```python
from build123d import *

# Parameters (mm, degrees)
BOSS_EXTRUDE1_DEPTH     = 5
BOSS_EXTRUDE2_DEPTH     = 7
SKETCH3_R               = 1.5
SKETCH3_W               = 8
SKETCH3_H               = 8
SKETCH3_R_2             = 2.5
BOSS_EXTRUDE3_DEPTH     = 5
SKETCH4_R               = 2.5
BOSS_EXTRUDE4_DEPTH     = 5
CUT_EXTRUDE1_DEPTH      = 123.769787834
CUT_EXTRUDE1_DEPTH_BACK = 123.769787834
SKETCH5_R               = 2.5
SKETCH5_R_2             = 2.55926668
SKETCH5_R_3             = 1.5
FILLET1_R               = 3.5


with BuildPart() as part:
    # Sketch1 → Boss-Extrude1 (new body)
    with BuildSketch(Plane(origin=(0, 0, 0), x_dir=(1, 0, 0), z_dir=(0, 1, 0))):
        Polygon((-57.597316241, 51.805869074), (-57.597316241, -8.444130926), (-46.097316241, -28.194130926), (-46.097316241, -108.194130926), (43.902683759, -108.194130926), (43.902683759, -28.194130926), (55.402683759, -8.444130926), (55.402683759, 51.805869074), align=None)
    extrude(amount=BOSS_EXTRUDE1_DEPTH)

    # Sketch2 → Boss-Extrude2 (add)
    with BuildSketch(Plane(origin=(0, 5, 0), x_dir=(1, 0, 0), z_dir=(0, 1, 0))):
        Polygon((-46.097316241, -28.194130926), (-46.097316241, -108.194130926), (43.902683759, -108.194130926), (43.902683759, -28.194130926), (41.402683759, -28.194130926), (41.402683759, -105.694130926), (-43.597316241, -105.694130926), (-43.597316241, -28.194130926), align=None)
        Polygon((52.902683759, -6.988434723), (55.402683759, -8.444130926), (43.902683759, -28.194130926), (41.402683759, -26.738434723), align=None)
        Polygon((41.402683759, -28.194130926), (43.902683759, -28.194130926), (41.402683759, -26.738434723), align=None)
        Polygon((52.902683759, -6.988434723), (55.402683759, -8.444130926), (55.402683759, -6.988434723), align=None)
        Polygon((-57.597316241, 51.805869074), (-57.597316241, -6.988434723), (-55.097316241, -6.988434723), (-55.097316241, 49.305869074), (52.902683759, 49.305869074), (52.902683759, -6.988434723), (55.402683759, -6.988434723), (55.402683759, 51.805869074), align=None)
        Polygon((-43.597316241, -26.738434723), (-46.097316241, -28.194130926), (-43.597316241, -28.194130926), align=None)
        Polygon((-43.597316241, -26.738434723), (-46.097316241, -28.194130926), (-57.597316241, -8.444130926), (-55.097316241, -6.988434723), align=None)
        Polygon((-57.597316241, -6.988434723), (-57.597316241, -8.444130926), (-55.097316241, -6.988434723), align=None)
    extrude(amount=BOSS_EXTRUDE2_DEPTH)

    # Sketch3 → Boss-Extrude3 (add)
    # profile 1 of 3: a face of its own
    with BuildSketch(Plane(origin=(0, 5, 0), x_dir=(1, 0, 0), z_dir=(0, 1, 0))):
        Polygon((-43.597316241, -99.694130926), (-43.597316241, -105.694130926), (41.402683759, -105.694130926), (41.402683759, -99.694130926), (32.902683759, -99.694130926), (20.902683759, -102.694130926), (-23.097316241, -102.694130926), (-35.097316241, -99.694130926), align=None)
        with Locations(Location((-39.347316241, -101.944130926, 0), (0, 0, 270))):
            Circle(SKETCH3_R, mode=Mode.SUBTRACT)
        with Locations(Location((37.152683759, -101.944130926, 0), (0, 0, 270))):
            Circle(SKETCH3_R, mode=Mode.SUBTRACT)
    # profile 2 of 3: a face of its own
    with BuildSketch(Plane(origin=(0, 5, 0), x_dir=(1, 0, 0), z_dir=(0, 1, 0))):
        with Locations((-51.097316241, 45.305869074)):
            Rectangle(SKETCH3_W, SKETCH3_H)
        with Locations(Location((-51.097316241, 45.305869074, 0), (0, 0, 270))):
            Circle(SKETCH3_R_2, mode=Mode.SUBTRACT)
    # profile 3 of 3: a face of its own
    with BuildSketch(Plane(origin=(0, 5, 0), x_dir=(1, 0, 0), z_dir=(0, 1, 0))):
        with Locations((48.902683759, 45.305869074)):
            Rectangle(SKETCH3_W, SKETCH3_H)
        with Locations(Location((48.902683759, 45.305869074, 0), (0, 0, 270))):
            Circle(SKETCH3_R_2, mode=Mode.SUBTRACT)
    extrude(amount=BOSS_EXTRUDE3_DEPTH)

    # Sketch4 → Boss-Extrude4 (add)
    # profile 1 of 2: a face of its own
    with BuildSketch(Plane(origin=(0, 5, 0), x_dir=(1, 0, 0), z_dir=(0, 1, 0))):
        Polygon((1.402683759, 10.130869074), (-55.097316241, 10.130869074), (-55.097316241, -6.988434723), (-43.597316241, -26.738434723), (-43.597316241, 0.130869074), (1.402683759, 0.130869074), align=None)
        with Locations(Location((-31.847316241, 5.130869074, 0), (0, 0, 90))):
            Circle(SKETCH4_R, mode=Mode.SUBTRACT)
        with Locations(Location((-21.847316241, 5.130869074, 0), (0, 0, 90))):
            Circle(SKETCH4_R, mode=Mode.SUBTRACT)
    # profile 2 of 2: a face of its own
    with BuildSketch(Plane(origin=(0, 5, 0), x_dir=(1, 0, 0), z_dir=(0, 1, 0))):
        Polygon((39.6145491, 10.130869074), (39.6145491, 0.130869074), (41.402683759, 0.130869074), (41.402683759, -26.738434723), (52.902683759, -6.988434723), (52.902683759, 10.130869074), align=None)
    extrude(amount=BOSS_EXTRUDE4_DEPTH)

    # Sketch5 → Cut-Extrude1 (cut, two sides: drawn at the far end of the back side and taken through both)
    with BuildSketch(Plane(origin=(0, 5, 0), x_dir=(1, 0, 0), z_dir=(0, 1, 0)).offset(-CUT_EXTRUDE1_DEPTH_BACK)):
        with Locations(Location((-21.847316241, 5.130869074, 0), (0, 0, 90))):
            Circle(SKETCH5_R)
        with Locations(Location((-31.847316241, 5.130869074, 0), (0, 0, 270))):
            Circle(SKETCH5_R_2)
        with Locations(Location((-39.347316241, -101.944130926, 0), (0, 0, 270))):
            Circle(SKETCH5_R_3)
        with Locations(Location((37.152683759, -101.944130926, 0), (0, 0, 270))):
            Circle(SKETCH5_R_3)
        with Locations(Location((-51.097316241, 45.305869074, 0), (0, 0, 270))):
            Circle(SKETCH5_R)
        with Locations(Location((48.902683759, 45.305869074, 0), (0, 0, 270))):
            Circle(SKETCH5_R)
        with Locations(Location((-49.597316241, -6.988434723, 0), (0, 0, 270))):
            Circle(SKETCH5_R)
        with Locations(Location((47.402683759, -6.988434723, 0), (0, 0, 270))):
            Circle(SKETCH5_R)
    extrude(amount=CUT_EXTRUDE1_DEPTH + CUT_EXTRUDE1_DEPTH_BACK, mode=Mode.SUBTRACT)

    # Fillet1
    # the kernel refuses this fillet: 3.5 mm, written as the material it adds along each edge
    with BuildSketch(Plane(origin=(41.402683759, 5, 99.694130926), x_dir=(0, 0, -1), z_dir=(0, 1, 0)), Plane(origin=(-55.097316241, 5, -41.305869074), x_dir=(0, 0, 1), z_dir=(0, 1, 0)), Plane(origin=(44.902683759, 5, -49.305869074), x_dir=(-1, 0, 0), z_dir=(0, 1, 0)), Plane(origin=(52.902683759, 5, -10.130869074), x_dir=(0, 0, -1), z_dir=(0, 1, 0)), Plane(origin=(-43.597316241, 5, -0.130869074), x_dir=(0, 0, 1), z_dir=(0, 1, 0))) as fillet1_piece_1:
        with BuildLine():
            CenterArc((FILLET1_R, FILLET1_R), FILLET1_R, 180, 90)
            Line((0, FILLET1_R), (0, 0))
            Line((0, 0), (FILLET1_R, 0))
        make_face()
    extrude(amount=5)
    with BuildSketch(Plane(origin=(20.902683759, 3.922825776, 102.694130926), x_dir=(-1, 0, 0), z_dir=(0, 1, 0)), Plane(origin=(-23.097316241, 3.922825776, 102.694130926), x_dir=(-0.9701425001453338, 0, -0.2425356250363252), z_dir=(0, 1, 0))) as fillet1_piece_2:
        with BuildLine():
            CenterArc((FILLET1_R * 0.123105625618, -FILLET1_R), FILLET1_R, 90, 14.036243468)
            Line((-FILLET1_R * 0.119429999419, -FILLET1_R * 0.0298574998547), (0, 0))
            Line((0, 0), (FILLET1_R * 0.123105625618, 0))
        make_face()
    extrude(amount=6.077174224)
    with BuildSketch(Plane(origin=(-43.597316241, 5, 99.694130926), x_dir=(0, 0, -1), z_dir=(0, 1, 0)), Plane(origin=(-47.097316241, 5, -49.305869074), x_dir=(1, 0, 0), z_dir=(0, 1, 0)), Plane(origin=(52.902683759, 5, -41.305869074), x_dir=(0, 0, 1), z_dir=(0, 1, 0)), Plane(origin=(-55.097316241, 5, -10.130869074), x_dir=(0, 0, -1), z_dir=(0, 1, 0))) as fillet1_piece_3:
        with BuildLine():
            CenterArc((FILLET1_R, -FILLET1_R), FILLET1_R, 90, 90)
            Line((0, -FILLET1_R), (0, 0))
            Line((0, 0), (FILLET1_R, 0))
        make_face()
    extrude(amount=5)
    with BuildSketch(Plane(origin=(43.902683759, 12, 28.194130926), x_dir=(0.5031907286678252, 0, -0.864175381842565), z_dir=(0, -1, 0)), Plane(origin=(-46.097316241, 0, 28.194130926), x_dir=(-0.5031907286678269, 0, -0.8641753818425641), z_dir=(0, 1, 0))) as fillet1_piece_4:
        with BuildLine():
            CenterArc((FILLET1_R * 0.269926710528, FILLET1_R), FILLET1_R, 239.788677614, 30.211322386)
            Line((-FILLET1_R * 0.23326401814, FILLET1_R * 0.135824618157), (0, 0))
            Line((0, 0), (FILLET1_R * 0.269926710528, 0))
        make_face()
    extrude(amount=12)
    with BuildSketch(Plane(origin=(41.402683759, 5, -0.130869074), x_dir=(0, 0, 1), z_dir=(0, 1, 0))) as fillet1_piece_5:
        with BuildLine():
            CenterArc((3.052788407, -3.5), FILLET1_R, 90, 60.718267745)
            Line((0, -1.788134659), (0, 0))
            Line((0, 0), (3.052788407, 0))
        make_face()
    extrude(amount=5)
    # the kernel refuses this fillet: 3.5 mm, written as the material it takes off along each edge
    with BuildSketch(Plane(origin=(32.902683759, 5, 99.694130926), x_dir=(1, 0, 0), z_dir=(0, 1, 0)), Plane(origin=(-35.097316241, 5, 99.694130926), x_dir=(0.9701425001453338, 0, 0.2425356250363252), z_dir=(0, 1, 0))) as fillet1_2_piece_1:
        with BuildLine():
            CenterArc((FILLET1_R * 0.123105625618, -FILLET1_R), FILLET1_R, 90, 14.036243468)
            Line((-FILLET1_R * 0.119429999419, -FILLET1_R * 0.0298574998547), (0, 0))
            Line((0, 0), (FILLET1_R * 0.123105625618, 0))
        make_face()
    extrude(amount=6.077174224, mode=Mode.SUBTRACT)
    with BuildSketch(Plane(origin=(-47.097316241, 5, -41.305869074), x_dir=(-1, 0, 0), z_dir=(0, 1, 0)), Plane(origin=(44.902683759, 5, -41.305869074), x_dir=(0, 0, -1), z_dir=(0, 1, 0)), Plane(origin=(39.6145491, 5, -10.130869074), x_dir=(1, 0, 0), z_dir=(0, 1, 0)), Plane(origin=(1.402683759, 5, -10.130869074), x_dir=(0, 0, 1), z_dir=(0, 1, 0))) as fillet1_2_piece_2:
        with BuildLine():
            CenterArc((FILLET1_R, -FILLET1_R), FILLET1_R, 90, 90)
            Line((0, -FILLET1_R), (0, 0))
            Line((0, 0), (FILLET1_R, 0))
        make_face()
    extrude(amount=13.75, mode=Mode.SUBTRACT)
    with BuildSketch(Plane(origin=(55.402683759, 14.361858717, 8.444130926), x_dir=(0, 0, -1), z_dir=(0, -1, 0)), Plane(origin=(-57.597316241, -2.361858717, 8.444130926), x_dir=(0, 0, -1), z_dir=(0, 1, 0))) as fillet1_2_piece_3:
        with BuildLine():
            CenterArc((FILLET1_R * 0.269926710528, -FILLET1_R), FILLET1_R, 90, 30.211322386)
            Line((-FILLET1_R * 0.23326401814, -FILLET1_R * 0.135824618157), (0, 0))
            Line((0, 0), (FILLET1_R * 0.269926710528, 0))
        make_face()
    extrude(amount=16.723717434, mode=Mode.SUBTRACT)
    with BuildSketch(Plane(origin=(43.902683759, 20.75, 108.194130926), x_dir=(-1, 0, 0), z_dir=(0, -1, 0))) as fillet1_2_piece_4:
        with BuildLine():
            CenterArc((FILLET1_R, FILLET1_R), FILLET1_R, 180, 90)
            Line((0, FILLET1_R), (0, 0))
            Line((0, 0), (FILLET1_R, 0))
        make_face()
    extrude(amount=29.5, mode=Mode.SUBTRACT)
    with BuildSketch(Plane(origin=(-46.097316241, -8.75, 108.194130926), x_dir=(0, 0, -1), z_dir=(0, 1, 0)), Plane(origin=(-57.597316241, -8.75, -51.805869074), x_dir=(1, 0, 0), z_dir=(0, 1, 0)), Plane(origin=(55.402683759, -8.75, -51.805869074), x_dir=(0, 0, 1), z_dir=(0, 1, 0))) as fillet1_2_piece_5:
        with BuildLine():
            CenterArc((FILLET1_R, -FILLET1_R), FILLET1_R, 90, 90)
            Line((0, -FILLET1_R), (0, 0))
            Line((0, 0), (FILLET1_R, 0))
        make_face()
    extrude(amount=29.5, mode=Mode.SUBTRACT)
    with BuildSketch(Plane(origin=(1.402683759, 5, -0.130869074), x_dir=(0, 0, -1), z_dir=(0, 1, 0))) as fillet1_2_piece_6:
        with BuildLine():
            CenterArc((FILLET1_R, FILLET1_R), FILLET1_R, 180, 90)
            Line((0, FILLET1_R), (0, 0))
            Line((0, 0), (FILLET1_R, 0))
        make_face()
    extrude(amount=13.75, mode=Mode.SUBTRACT)


solid = part.part
```
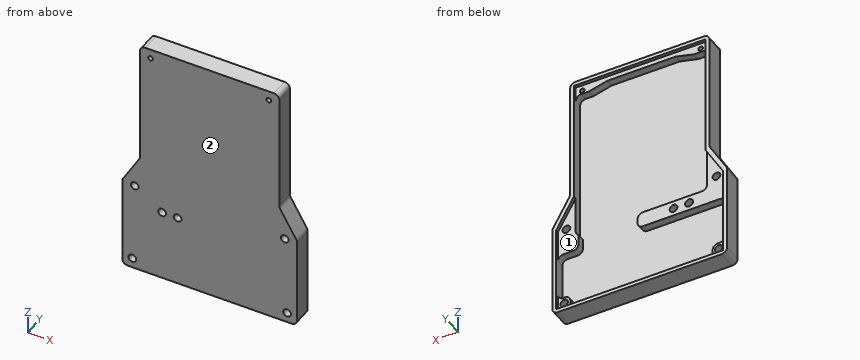
Input: part model. Units: mm. Frame: model coordinates. Face numbers are marked on the shaded views. Coordinates: 2 decimals unless noted, no trailing zeros. Loops run counter-clockwise (first coordinate to the right, second up) from the corner with the lowest first, then second, coordinate; pieces in that order, holes last. Notation, with made-up numbers: M -14,16.5 L 41,16.5 A21 cw 41,46.5 Z; hole C 77,-18 d4. An arc over 180 degrees is marked long. Use a Markdown table: item, result. Add a question column.
1) Section C-C, the plane z = 24.5. Return the cut outline in (x, y), plus the area to 3 significant figures.
2) Section B-B, the plane z = 73.5. Return the cut outline in (x, y).
3) Pin query (flat end, axial travel): P1, Ø5, axis at x = -8, z = 98.5, coming from the +Y side; P2, Ø1, axis at y = 3, z = 24, coming from the -X side; P3, Ø3.5, axis at x = 37.15, z = 101.94, coming from the +Y side; P4, Ø4.5, axis at x = -51.1, z = -45.31, coming from the +Y side. Return the tip coordinate at first contact, or that it passes through.
4) Section A-A, the plane y = 1.75. Give the number of separate pieces and of enclosed holes in the cut face, plus the area to 3 significant figures.
5) Draft query along X for the marked faces 1 and 2. Return one class per face: +X half, -X half, draft (parallel to the pull), parting line (faces both ways), or undercut.
6) Line query: L1, parallel to X at y = 6, z = -22.5; L2, parallel to X at y = 5.75, z = 39; L3, parallel to Z at x = 50.5, y = 7.25. Output: solid intervals per line, ascending. Write a range as from..to.
Answer below:
| question | item | result |
|---|---|---|
| 1 | outline | M -48.25,0 L 46.05,0 L 46.05,12 L 42.71,12 L 42.71,10 L 41.4,10 L 41.4,5 L -43.6,5 L -43.6,10 L -44.9,10 L -44.9,12 L -48.25,12 Z |
| 1 | area | 531 mm2 |
| 2 | outline | M -46.1,0 L 43.9,0 L 43.9,12 L 41.4,12 L 41.4,5 L -43.6,5 L -43.6,12 L -46.1,12 Z |
| 3 | P1 | y = 5 |
| 3 | P2 | x = -48.83 |
| 3 | P3 | y = 10 |
| 3 | P4 | through |
| 4 | separate pieces | 1 |
| 4 | enclosed holes | 8 |
| 4 | area | 15,900 mm2 |
| 5 | face 1 | undercut |
| 5 | face 2 | draft |
| 6 | L1 | -57.6..-55.1, 52.9..55.4 |
| 6 | L2 | -46.1..-43.6, 41.4..43.9 |
| 6 | L3 | -51.81..-47.23, -43.38..-41.13, -10.31..16.86 |
